Autodesk Inventor part; units mm, degrees
ref_plane "YZ Plane" through (0, 0, 0) normal (1, 0, 0) x (0, 1, 0)
ref_plane "XZ Plane" through (0, 0, 0) normal (0, 1, 0) x (-1, 0, 0)
ref_plane "XY Plane" through (0, 0, 0) normal (0, 0, 1) x (1, 0, 0)
sketch "Schizzo1" plane through (0, 0, 0) normal (0, 0, 1) x (1, 0, 0)
  line L0 (37.5, -42.5) -> (-37.5, -42.5)
  line L1 (-42.5, -37.5) -> (-42.5, 37.5)
  line L2 (-37.5, 42.5) -> (37.5, 42.5)
  line L3 (42.5, 37.5) -> (42.5, -37.5)
  line L4 (42.5, -42.5) -> (-42.5, 42.5) construction
  line L5 (-42.5, -42.5) -> (42.5, 42.5) construction
  arc A0 (-42.5, -37.5) -> (-37.5, -42.5) centre (-37.5, -37.5) ccw
  line L6 (-42.5, 42.5) -> (42.5, -42.5) construction
  arc A1 (-37.5, 42.5) -> (-42.5, 37.5) centre (-37.5, 37.5) ccw
  arc A2 (37.5, -42.5) -> (42.5, -37.5) centre (37.5, -37.5) ccw
  arc A3 (42.5, 37.5) -> (37.5, 42.5) centre (37.5, 37.5) ccw
  circle A4 centre (-34, -34) radius 5.2
  circle A5 centre (-34, 34) radius 5.2
  circle A6 centre (34, -34) radius 5.2
  circle A7 centre (34, 34) radius 5.2
  circle A8 centre (0, 0) radius 12
  circle A9 centre (0, 0) radius 20
  dimension "d12" = 85
  dimension "d17" = 10.4
  dimension "d18" = 24
  dimension "d19" = 40
extrude "Estrusione1" add sketch "Schizzo1" along normal mid plane 8 contours L0 A0 L1 A1 L2 A3 L3 A2
sketch "Schizzo2" plane through (0, 0, -4) normal (0, 0, -1) x (-1, 0, 0)
  circle A0 centre (-34, 34) radius 5.2
  circle A1 centre (-34, 34) radius 5.2
  circle A2 centre (-34, 34) radius 2.5
  line L0 (-37.5, 42.5) -> (37.5, 42.5)
  line L1 (0, 42.5) -> (0, -42.5)
  line L2 (-37.5, -42.5) -> (37.5, -42.5)
  line L3 (-42.5, -37.5) -> (-42.5, 37.5)
  line L4 (-42.5, 0) -> (42.5, 0)
  line L5 (42.5, 37.5) -> (42.5, -37.5)
  circle A3 centre (34, 34) radius 5.2
  circle A4 centre (34, 34) radius 2.5
  circle A5 centre (-34, -34) radius 5.2
  circle A6 centre (-34, -34) radius 2.5
  circle A7 centre (34, -34) radius 2.5
  circle A8 centre (34, -34) radius 5.2
  point P0 (0, 0)
  dimension "d22" = 5
extrude "Estrusione2" add sketch "Schizzo2" against normal blind 8 contours A3
mirror "Speculare1" about plane through (0, 0, 0) normal (1, 0, 0) of "Estrusione2"
mirror "Speculare2" about plane through (0, 0, 0) normal (0, 1, 0) of "Estrusione2", "Speculare1"
sketch "Schizzo3" plane through (0, 0, -4) normal (0, 0, -1) x (-1, 0, 0)
  line L0 (37.5, -42.5) -> (-37.5, -42.5)
  line L1 (0, -42.5) -> (0, -40.5)
  line L2 (-37.5, -40.5) -> (37.5, -40.5)
  line L3 (-42.5, -37.5) -> (-42.5, 37.5)
  line L4 (-42.5, 0) -> (42.5, 0)
  line L5 (42.5, 37.5) -> (42.5, -37.5)
  line L6 (0, -42.5) -> (0, 42.5)
  line L7 (-37.5, 42.5) -> (37.5, 42.5)
  line L8 (-37.5, 40.5) -> (37.5, 40.5)
  line L9 (-42.5, 0) -> (-40.5, 0)
  line L10 (-40.5, -37.5) -> (-40.5, 37.5)
  line L11 (40.5, -37.5) -> (40.5, 37.5)
  arc A0 (37.5, -40.5) -> (40.5, -37.5) centre (37.5, -37.5) ccw
  arc A1 (-40.5, -37.5) -> (-37.5, -40.5) centre (-37.5, -37.5) ccw
  arc A2 (40.5, 37.5) -> (37.5, 40.5) centre (37.5, 37.5) ccw
  arc A3 (-37.5, 40.5) -> (-40.5, 37.5) centre (-37.5, 37.5) ccw
  circle A4 centre (0, 0) radius 20
  circle A5 centre (0, 0) radius 25
  dimension "d25" = 2
  dimension "d27" = 2
extrude "Estrusione3" cut sketch "Schizzo3" against normal blind 1 contours A1 L10 L4 A5 L6 L2 | L6 A5 L4 L11 A0 L2 | L10 A3 L8 L6 A5 L4 | A5 L6 L8 A2 L11 L4
sketch "Schizzo4" plane through (0, 0, -3) normal (0, 0, -1) x (-1, 0, 0)
  line L0 (37.5, -40.5) -> (-37.5, -40.5)
  line L1 (0, -40.5) -> (0, -38.5)
  line L2 (-37.5, -38.5) -> (37.5, -38.5)
  line L3 (-42.5, 37.5) -> (-42.5, -37.5)
  line L4 (-37.5, -42.5) -> (37.5, -42.5)
  line L5 (37.5, 42.5) -> (-37.5, 42.5)
  line L6 (-37.5, 38.5) -> (37.5, 38.5)
  line L7 (-38.4396, 0) -> (-0.9396, 0) construction
  line L8 (-40.5, -37.5) -> (-40.5, 37.5)
  line L9 (-40.5, 0) -> (-38.5, 0)
  line L10 (-38.5, -37.5) -> (-38.5, 37.5)
  arc A0 (-37.5, 38.5) -> (-38.5, 37.5) centre (-37.5, 37.5) ccw
  line L11 (38.5, -37.5) -> (38.5, 37.5)
  arc A1 (38.5, 37.5) -> (37.5, 38.5) centre (37.5, 37.5) ccw
  arc A2 (-38.5, -37.5) -> (-37.5, -38.5) centre (-37.5, -37.5) ccw
  arc A3 (37.5, -38.5) -> (38.5, -37.5) centre (37.5, -37.5) ccw
  point P0 (0, 0)
  dimension "d31" = 2
  dimension "d35" = 2
  dimension "d36" = 75
extrude "Estrusione4" cut sketch "Schizzo4" against normal blind 1.5 from surface at 0
sketch "Schizzo5" plane through (37.5, -38.5, -1.5) normal (0, 0, -1) x (-1, 0, 0)
  circle A0 centre (3.5, 4.5) radius 2.5
  circle A1 centre (3.5, 4.5) radius 2.5
  point P0 (37.5, 38.5)
hole "Foro1" at (34, -34, -1.5) direction (0, 0, 1) diameter 5.5 end through all countersink diameter 10.4 countersink angle 90
mirror "Speculare3" about plane through (0, 0, 0) normal (1, 0, 0) of "Foro1"
mirror "Speculare4" about plane through (0, 0, 0) normal (0, 1, 0) of "Foro1", "Speculare3"
sketch "Schizzo6" plane through (31.3942, -38.5, -1.5) normal (0, 0, -1) x (-1, 0, 0)
  line L0 (62.7885, 0) -> (0, 0)
  line L1 (31.3942, 0) -> (31.3942, 3)
  line L2 (31.3942, 3) -> (57.3377, 3)
  line L3 (31.3942, 3) -> (5.4507, 3)
  line L4 (-7.1058, 1) -> (-7.1058, 76)
  line L5 (-7.1058, 38.5) -> (-4.1058, 38.5)
  line L6 (-4.1058, 38.5) -> (-4.1058, 64.4435)
  line L7 (-4.1058, 38.5) -> (-4.1058, 12.5565)
  line L8 (-11.1058, 1) -> (-11.1058, 76)
  line L9 (-11.1058, 38.5) -> (73.8942, 38.5)
  line L10 (73.8942, 76) -> (73.8942, 1)
  line L11 (31.3942, -3.9455) -> (31.3942, 81)
  line L12 (-6.1058, 81) -> (68.8942, 81)
  line L13 (31.3942, 74) -> (57.3377, 74)
  line L14 (31.3942, 74) -> (5.4507, 74)
  line L15 (66.8942, 38.5) -> (66.8942, 64.4435)
  line L16 (66.8942, 38.5) -> (66.8942, 12.5565)
  arc A0 (66.8942, 12.5565) -> (57.3377, 3) centre (66.8942, 3) ccw
  arc A1 (57.3377, 74) -> (66.8942, 64.4435) centre (66.8942, 74) ccw
  arc A2 (5.4507, 3) -> (-4.1058, 12.5565) centre (-4.1058, 3) ccw
  arc A3 (-4.1058, 64.4435) -> (5.4507, 74) centre (-4.1058, 74) ccw
  point P0 (31.3942, 38.5)
  dimension "d46" = 3
  dimension "d47" = 25.9435
  dimension "d48" = 25.9435
  dimension "d49" = 3
  dimension "d51" = 25.9435
extrude "Estrusione5" cut sketch "Schizzo6" against normal blind 1
sketch "Schizzo8" plane through (0, 0, -4) normal (0, 0, -1) x (-1, 0, 0)
  line L0 (-1, 21.321) -> (1, 21.321)
  line L1 (1, 21.321) -> (1, 18.679)
  line L2 (1, 18.679) -> (-1, 18.679)
  line L3 (-1, 18.679) -> (-1, 21.321)
  circle A0 centre (0, 0) radius 20
  line L4 (-1, 21.321) -> (1, 18.679) construction
  line L5 (1, 21.321) -> (-1, 18.679) construction
  point P0 (0, 20)
  point P1 (1, 19.975)
  point P2 (-1, 19.975)
  dimension "d54" = 2
  dimension "d55" = 2.642
sketch "Schizzo9" plane through (0, 0, -3) normal (0, 0, 1) x (1, 0, 0)
  circle A0 centre (0, 0) radius 25
  circle A1 centre (0, 0) radius 20
  dimension "d56" = 50
extrude "Estrusione6" add sketch "Schizzo9" along normal blind 2.7
extrude "Estrusione7" add sketch "Schizzo8" against normal blind 8 contours A0 L1 L2 L3 picked at (0.1112, 19.1184)
pattern_circular "Serie circolare1" count 4 over 360 about axis through (0, 0, 0) along (0, 0, 1) of "Estrusione7"
CAD build for the part. Positions are in the model's coordinates, mm. A direction names the side the tool comes from. Coordinates: 2 decimals unless noted, no trailing zeros. Write each loop counter-clockwise with the first axis right and the second up, starting at its lowest first coordinate (ties: lowest second). Pieces come first, ordered by that corner, then holes. Notation, with made-up numbers: (66, 34.5) - (103, 34.5) arc R38 cw to (103, 72.5) - close; hole circle Ø7 at (-35.5, -6.75). An arc over 180 degrees is marked (long way). Use a Markdown table: item, result. Add a question column.
Item 1: Band-saw the part on A-A, the plane y = 0. Give the cut face in (x, z).
Item 2: Flat gauge pins, fed straight in: pin 1 (6 mm diameter, centred on x = -23, y = -28, fed in from -Z); pin 2 (2 mm diameter, centred on x = 27.5, y = 32, fed in from -Z); pin 3 (7 mm diameter, centred on x = -34, y = -34, fed in from -Z); pin 4 (6.5 mm diameter, centred on x = 34, y = 34, fed in from +Z). Where does each tip first touch, or does it go through?
Item 3: Band-saw the part on D-D, the plane y = 34. Give the cut face in (x, z), and give its area (3 significant figures).
Item 4: Band-saw the part on C-C, the plane z = 2.25. Give the cut face in (x, y), and give its area (3 significant figures).
Item 5: 3-axis set-ups, long thin cutter, end or side, ignore diameter. For faces 1 (the face through (39.64, -39.6, -3.51)), 2 (the face through (-18.679, 0, 0)), 3 (the face through (-1, 42.5, 0)): which of +Z, -Z, +X, -X, +Y, -Y reach the whole face in a straight line?
Item 6: Drill centre lines: L1, parallel to X at y = 34, z = 1.8; L2, parallel to X at y = -8, z = -1.75. Where is each one in solid material? Low to high. Write a range as from..to.
Item 7: Mould opens along X. For faces 4 (the face through (-39.6, -39.64, -3.51)), 5 (the face through (19.5, 0.6, 4)), 6 (the face through (3, -39, -3)), 7 (the face through (42.5, 1, 0)) say: pulls with the +X half, pulls with the -X half, needs draft (parallel to the pull), parting line crosses it, or undercut.
Numbers:
| question | item | result |
|---|---|---|
| 1 | outline | (-42.5, -4) - (-40.5, -4) - (-40.5, -3) - (-38.5, -3) - (-38.5, -1.5) - (-35.5, -1.5) - (-35.5, -0.5) - (-25, -0.5) - (-25, -4) - (-18.68, -4) - (-18.68, 4) - (-42.5, 4) - close; (18.68, -4) - (25, -4) - (25, -0.5) - (35.5, -0.5) - (35.5, -1.5) - (38.5, -1.5) - (38.5, -3) - (40.5, -3) - (40.5, -4) - (42.5, -4) - (42.5, 4) - (18.68, 4) - close |
| 2 | pin 1 | z = -0.5 |
| 2 | pin 2 | z = -1.5 |
| 2 | pin 3 | z = 0.2 |
| 2 | pin 4 | z = 4 |
| 3 | outline | (-42.5, -4) - (-40.5, -4) - (-40.5, -3) - (-38.5, -3) - (-38.5, -1.5) - (-39.2, -1.5) - (-36.75, 0.95) - (-36.75, 4) - (-42.5, 4) - close; (-31.25, 0.95) - (-28.8, -1.5) - (-26.06, -1.5) - (-26.06, -0.5) - (26.06, -0.5) - (26.06, -1.5) - (28.8, -1.5) - (31.25, 0.95) - (31.25, 4) - (-31.25, 4) - close; (36.75, 0.95) - (39.2, -1.5) - (38.5, -1.5) - (38.5, -3) - (40.5, -3) - (40.5, -4) - (42.5, -4) - (42.5, 4) - (36.75, 4) - close |
| 3 | area | 359 mm2 |
| 4 | outline | (-42.5, -37.5) arc R5 ccw to (-37.5, -42.5) - (37.5, -42.5) arc R5 ccw to (42.5, -37.5) - (42.5, 37.5) arc R5 ccw to (37.5, 42.5) - (-37.5, 42.5) arc R5 ccw to (-42.5, 37.5) - close; hole circle Ø5.5 at (-34, -34); hole circle Ø5.5 at (-34, 34); hole (-19.97, -1) arc R20 ccw to (-1, -19.97) - (-1, -18.68) - (1, -18.68) - (1, -19.97) arc R20 ccw to (19.97, -1) - (18.68, -1) - (18.68, 1) - (19.97, 1) arc R20 ccw to (1, 19.97) - (1, 18.68) - (-1, 18.68) - (-1, 19.97) arc R20 ccw to (-19.97, 1) - (-18.68, 1) - (-18.68, -1) - close; hole circle Ø5.5 at (34, -34); hole circle Ø5.5 at (34, 34) |
| 4 | area | 5,860 mm2 |
| 5 | face 1 | -Z |
| 5 | face 2 | +Z, -Z |
| 5 | face 3 | +Z, -Z, +X, -X, +Y |
| 6 | L1 | -42.5..-36.75, -31.25..31.25, 36.75..42.5 |
| 6 | L2 | -42.5..-38.5, -23.69..-18.33, 18.33..23.69, 38.5..42.5 |
| 7 | face 4 | undercut |
| 7 | face 5 | needs draft |
| 7 | face 6 | undercut |
| 7 | face 7 | pulls with the +X half |
